The listing builds one solid part. Answer for the finished solid, in the listing's coordinates (mm). A direction names the side the tool comes from. Coordinates: 2 decimals unless noted, no trailing zeros. Loops run counter-clockwise (first coordinate to the right, second up) from the corner with the lowest first, then second, coordinate; pieces in that order, holes last. Notation, with made-up numbers: (79.25, 59) - (93.25, 59) arc R23 cw to (93.25, 95) - close; hole circle Ø10 at (32, 44.5). An arc over 180 degrees is marked (long way). Write each question's results on one line, items separated by ' | '. Start each with the question number.
(1) For faces 1 (the flat face through (-14.65, -1, 14)), 2 (the flat face through (-19.65, -1, 10)), 3 (the flat face through (-6, -1, 4.08)), 4 (the flat face through (-2.65, -1, 2)), 5 (the cylindrical face through (-12.237, -12.167, 1.972)), determine the directions among +Z, -Z, +X, -X, +Y, -Y from which every point of the face is accessible in a straight line to the end or side of a thin tool.
(2) Given pin 1 Ø5 at (y, z) = (4, 15.5) entering from +X; pin 2 Ø8 at (x, y) = (-4.5, -8.5) entering from +Z; pin 3 Ø1 at (x, y) = (3.5, -5.5) entering from -Z; pin 4 Ø2 at (x, y) = (-11, -10.5) entering from -Z, each flat-ended and moving along its own axis, determine where each tip first touches the part or whether it passes through.
(3) Find section A-A on z = 7.75. Determine the outline of the cut face in (x, y).
(4) Consider line 1 (X direction, y = -10.75, z = 1.75); line 2 (Z direction, x = -1, y = 6); line 3 (Z direction, x = 16.5, y = -9). Determine where each line is inside the solid, lowest interval first. Write a range as from..to.
(5) Find section D-D on y = -10. Determine the outline of the cut face in (x, z).
(6) Find section C-C on y = -3.75. Determine the outline of the cut face in (x, z).
(7) Determine the mould class of faces 6 (the flat face through (4, -6.95, 4)), 7 (the flat face through (3, 6, 8.2)), 8 (the flat face through (0, -14.95, 5)) for opening direction Y: released by +Y, released by -Y, zero draft, split by the parting line, or undercut.
(8) Find section B-B on x = 2.5. Determine the outline of the cut face in (y, z).
from build123d import *

# Parameters (mm, degrees)
F0_W     = 35.4
F0_H     = 28.5
F0_R     = 2
F1_DEPTH = 8.2
F0_W_2   = 5
F2_DEPTH = 20
F0_W_3   = 7.2
F0_H_2   = 12.5
F3_DEPTH = 4.08
F4_DEPTH = 4


with BuildPart() as f1:
    # F0 (on Top) → F1 (new body)
    with BuildSketch(Plane.XY):
        with Locations((3.049638, -0.700136)):
            Rectangle(F0_W, F0_H)
        with Locations((-10.650362, -10.950136)):
            Circle(F0_R, mode=Mode.SUBTRACT)
        with Locations((16.749638, -10.950136)):
            Circle(F0_R, mode=Mode.SUBTRACT)
        with Locations((-10.650362, 9.549864)):
            Circle(F0_R, mode=Mode.SUBTRACT)
        Polygon((-9.850362, -6.950136), (-9.850362, 5.549864), (-2.650362, 5.549864), (12.749638, 5.549864), (12.749638, -6.950136), (-2.650362, -6.950136), align=None, mode=Mode.SUBTRACT)
        with Locations((16.749638, 9.549864)):
            Circle(F0_R, mode=Mode.SUBTRACT)
        with Locations((-10.650362, 9.549864)):
            Circle(F0_R)
        with Locations((16.749638, 9.549864)):
            Circle(F0_R)
        with Locations((16.749638, -10.950136)):
            Circle(F0_R)
        with Locations((-10.650362, -10.950136)):
            Circle(F0_R)
    extrude(amount=F1_DEPTH)

    # F0 (on Top) → F2 (join)
    with BuildSketch(Plane.XY):
        with Locations((-17.150362, -0.700136)):
            Rectangle(F0_W_2, F0_H)
    extrude(amount=F2_DEPTH)

    # F0 (on Top) → F3 (join)
    with BuildSketch(Plane.XY):
        with Locations((-6.250362, -0.700136)):
            Rectangle(F0_W_3, F0_H_2)
    extrude(amount=F3_DEPTH)

    # F0 (on Top) → F4 (cut)
    with BuildSketch(Plane.XY):
        with Locations((-10.650362, -10.950136)):
            Circle(F0_R)
        with Locations((16.749638, -10.950136)):
            Circle(F0_R)
        with Locations((16.749638, 9.549864)):
            Circle(F0_R)
        with Locations((-10.650362, 9.549864)):
            Circle(F0_R)
    extrude(amount=F4_DEPTH, mode=Mode.SUBTRACT)


solid = f1.part
Values:
1) face 1: +Z, +X, +Y, -Y | face 2: +Z, -Z, -X, +Y, -Y | face 3: +Z | face 4: +Z, -Z | face 5: -Z
2) pin 1: stops at x = -14.65 | pin 2: stops at z = 8.2 | pin 3: passes through | pin 4: stops at z = 4
3) outline: (-19.65, -14.95) - (20.75, -14.95) - (20.75, 13.55) - (-19.65, 13.55) - close; hole (-9.85, -6.95) - (12.75, -6.95) - (12.75, 5.55) - (-9.85, 5.55) - close
4) line 1: x = -19.65..-12.64, -8.66..14.76, 18.74..20.75 | line 2: z = 0..8.2 | line 3: z = 4..8.2
5) outline: (-19.65, 0) - (-12.41, 0) - (-12.41, 4) - (-8.89, 4) - (-8.89, 0) - (14.99, 0) - (14.99, 4) - (18.51, 4) - (18.51, 0) - (20.75, 0) - (20.75, 8.2) - (-14.65, 8.2) - (-14.65, 20) - (-19.65, 20) - close
6) outline: (-19.65, 0) - (-2.65, 0) - (-2.65, 4.08) - (-9.85, 4.08) - (-9.85, 8.2) - (-14.65, 8.2) - (-14.65, 20) - (-19.65, 20) - close; (12.75, 0) - (20.75, 0) - (20.75, 8.2) - (12.75, 8.2) - close
7) face 6: undercut | face 7: zero draft | face 8: released by -Y
8) outline: (-14.95, 0) - (-6.95, 0) - (-6.95, 8.2) - (-14.95, 8.2) - close; (5.55, 0) - (13.55, 0) - (13.55, 8.2) - (5.55, 8.2) - close
